Design review of the part built by this model. Coordinates are the model's own, in mm. A direction names the side the tool comes from. Coordinates: 2 decimals unless noted, no trailing zeros. Write each loop counter-clockwise with the first axis right and the second up, starting at its lowest first coordinate (ties: lowest second). Pieces come first, ordered by that corner, then holes. Notation, with made-up numbers: (35.5, -7.75) -> (59.5, -7.75) arc R21 cw to (59.5, -3.75) -> close; hole circle Ø3 at (61, -5.75). An arc over 180 degrees is marked (long way). Answer in a Markdown table with one row per item. Add a question column.
Item 1: To check wall thickness, follow line 1 (Y direction, x = -40.5, z = -17.5); line 2 (Z direction, x = -2, y = -12); line 3 (X direction, y = 37.5, z = 6). State the ranges of each line that lie inside material, in increasing order.
Item 2: Draft analysis for pull direction Y (two halves, no side actions). For faces 1 (the face through (0, -30, 0)), 2 (the face through (11.923, -14.79, -3.755)), 3 (the face through (0, 50, 0)), state which applies: released by +Y, released by -Y, zero draft, split by the parting line, or undercut.
Item 3: Take a section at D-D, the plane x = 40. Write out the cut boundary in (y, z).
Item 4: Take a section at A-A, the plane z = 0. Write out the cut boundary in (x, y), and give its area (3 significant figures).
Item 5: Clearance check with flat-ended pins moving along their axes: P1, Ø6, axis at x = 11, z = -22, coming from the -Y side; P2, Ø2, axis at x = -9.5, y = 40.5, coming from the +Z side; P3, Ø4, axis at y = -3.5, z = -9, coming from the -X side. State where each tip first meets the part, or that it passes through.
Item 6: Take a section at B-B, the plane x = 0. Write out the cut boundary in (y, z), and give its area (3 significant figures).
Item 7: Take a section at C-C, the plane y = 4. Write out the cut boundary in (x, z), and give its area (3 significant figures).
Item 8: For faces 4 (the face through (10, 0, 10)), 5 (the face through (11.923, 34.79, -3.755)), 6 (the face through (47.69, 9.86, -15.02)), list the 3-axis set-ups (+Z, -Z, +X, -X, +Y, -Y) from which the entire face can be reached by the end or side of a thin tool; tool diameter is ignored.
from build123d import *

# Parameters (mm, degrees)
ESBO_O2_R                     = 50
RESSALTO_EXTRUS_O1_DEPTH      = 20
ESBO_O3_R                     = 12.5
RESSALTO_EXTRUS_O2_DEPTH      = 40
RESSALTO_EXTRUS_O2_DEPTH_BACK = 40


with BuildPart() as part:
    # Esboço2 → Ressalto-extrusão1 (new body)
    with BuildSketch(Plane(origin=(0, 0, 0), x_dir=(1, 0, 0), z_dir=(0, 1, 0))):
        Circle(ESBO_O2_R)
    extrude(amount=RESSALTO_EXTRUS_O1_DEPTH)

    # Esboço3 → Ressalto-extrusão2 (add, two sides)
    with BuildSketch(Plane(origin=(0, 10, 0), x_dir=(1, 0, 0), z_dir=(0, 1, 0))) as ressalto_extrus_o2_sk:
        Circle(ESBO_O3_R)
    extrude(amount=RESSALTO_EXTRUS_O2_DEPTH)
    extrude(ressalto_extrus_o2_sk.sketch, amount=-RESSALTO_EXTRUS_O2_DEPTH_BACK)


solid = part.part
Answers:
| question | item | result |
|---|---|---|
| 1 | line 1 | y = 0 to 20 |
| 1 | line 2 | z = -12.34 to 12.34 |
| 1 | line 3 | x = -10.97 to 10.97 |
| 2 | face 1 | released by -Y |
| 2 | face 2 | zero draft |
| 2 | face 3 | released by +Y |
| 3 | outline | (0, -30) -> (20, -30) -> (20, 30) -> (0, 30) -> close |
| 4 | outline | (-50, 0) -> (-12.5, 0) -> (-12.5, -30) -> (12.5, -30) -> (12.5, 0) -> (50, 0) -> (50, 20) -> (12.5, 20) -> (12.5, 50) -> (-12.5, 50) -> (-12.5, 20) -> (-50, 20) -> close |
| 4 | area | 3,500 mm^2 |
| 5 | P1 | stops at y = 0 |
| 5 | P2 | stops at z = 9.17 |
| 5 | P3 | stops at x = -10.36 |
| 6 | outline | (-30, -12.5) -> (0, -12.5) -> (0, -50) -> (20, -50) -> (20, -12.5) -> (50, -12.5) -> (50, 12.5) -> (20, 12.5) -> (20, 50) -> (0, 50) -> (0, 12.5) -> (-30, 12.5) -> close |
| 6 | area | 3,500 mm^2 |
| 7 | outline | circle Ø100 at (0, 0) |
| 7 | area | 7,850 mm^2 |
| 8 | face 4 | -Y |
| 8 | face 5 | +Y |
| 8 | face 6 | +Y, -Y |
